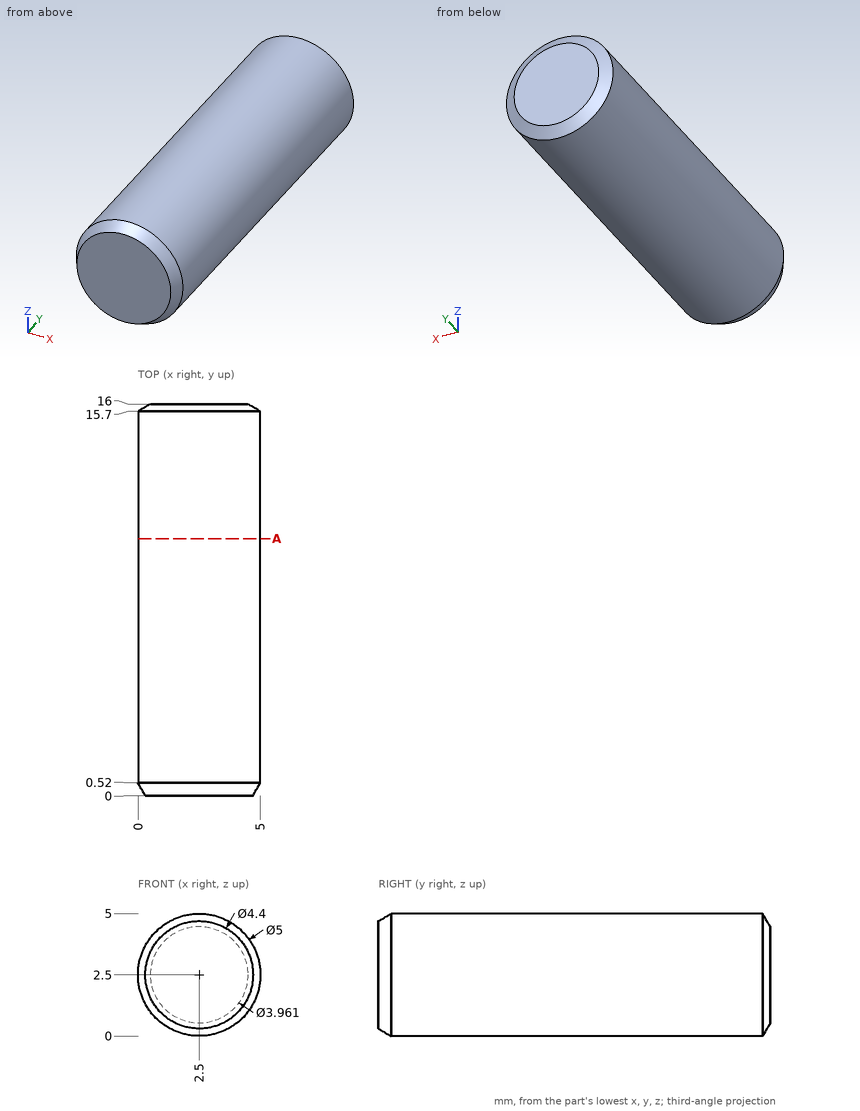
Geometry check sheet. Reference: drawing and pictorial views, mm from the part's lowest x, y, z. Round coordinates to 2 decimals unless told otherwise and drop trailing zeros. Loops run counter-clockwise (first coordinate to the right, second up) from the corner with the lowest first, then second, coordinate; pieces in that order, holes last. Notation, with made-up numbers: (43.25, -14.75) - (70.25, -14.75) arc R36 cw to (70.25, 19.25) - close; hole circle Ø4 at (68, 65.25). An arc over 180 degrees is marked (long way). Answer in a Markdown table with one row per item. Add a question column.
Q1. Material ranges on line 1 (Y direction, x = 1.2, z = 4.3) (1 decimal); line 2 (X direction, y = 10.25, z = 0.6) (1 decimal); line 3 (Y direction, x = 0.6, z = 1.85) (1 decimal), recorded low to high.
Q2. Gauge pin test, flat end, axial feed: pin 1 (1 mm diameter, centred on y = 8.5, z = 3.5, fed in from -X). Record the tip position at first contact, or that the pin passes through.
Q3. Section check A-A on y = 10.5. Enter the section's corners in (x, z), plus the area to 3 significant figures.
Found:
| question | item | result |
|---|---|---|
| 1 | line 1 | y = 0 to 15.9 |
| 1 | line 2 | x = 0.9 to 4.1 |
| 1 | line 3 | y = 0 to 16 |
| 2 | pin 1 | stops at x = 0.05 |
| 3 | outline | circle Ø5 at (2.5, 2.5) |
| 3 | area | 19.6 mm² |
